Part print with two shaded views. Sizes in mm from the minimum x, y, z corner. A direction names the side the tool comes from. Round coordinates to 2 decimals unless told otherwise and drop trailing zeros. Loops run counter-clockwise (first coordinate to the right, second up) from the corner with the lowest first, then second, coordinate; pieces in that order, holes last. Notation, with made-up numbers: (-13.5, -4) -> (9.5, -4) arc R13 ccw to (9.5, 19) -> close; hole circle Ø9 at (54, -26.5). An arc over 180 degrees is marked (long way). Put each result on its own line as item: value. Start each with the question number.
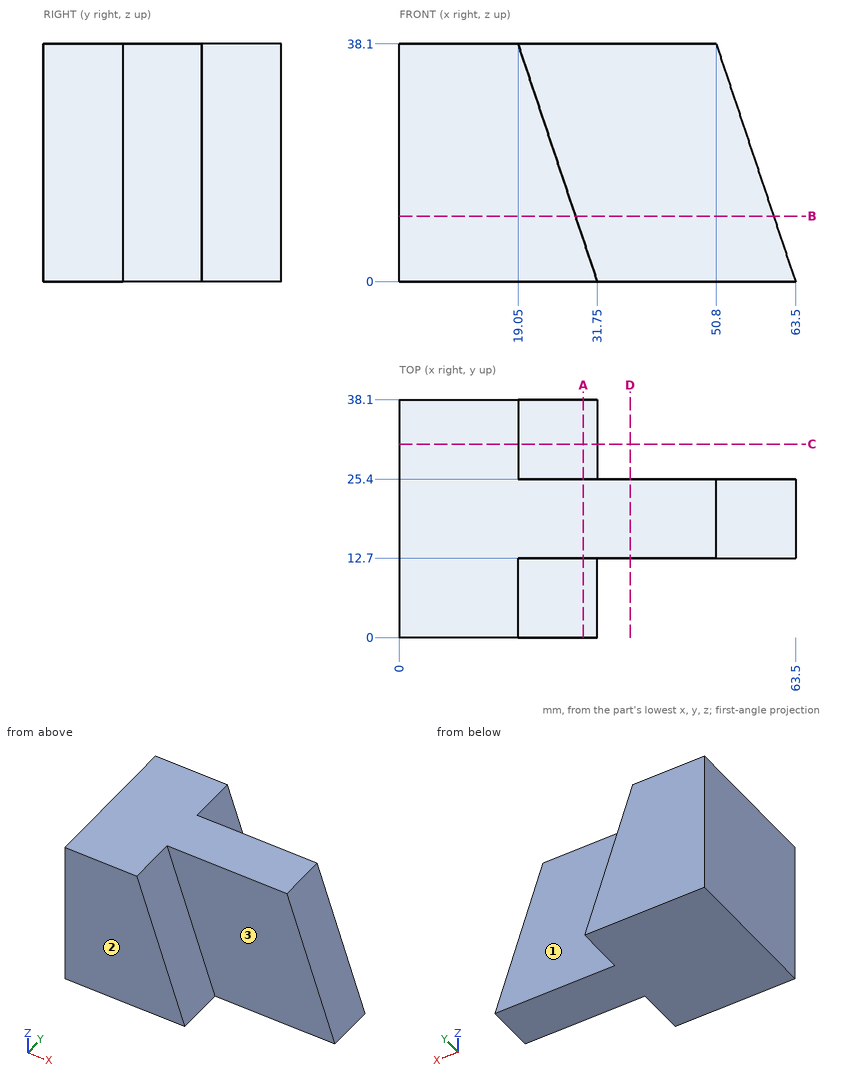
Item 1: Drop a flat-ended pin along its axis: pin 1 (2 mm diameter, centred on x = 40, z = 19.5, fed in from -Y). Give the stop position or say it passes through.
Item 2: Cut at A-A on x = 29.5. Write the cut outline in (y, z).
Item 3: Wall check: line 1 (Y direction, x = 48.5, z = 12.5); line 2 (X direction, y = 17.5, z = 25.5); line 3 (X direction, y = 16.5, z = 20). Give the ranges that are in metal, low to high. Write a range as from..to.
Item 4: 3-axis set-ups, long thin cutter, end or side, ignore diameter. For the marked faces 1, 2 and 3: which of +Z, -Z, +X, -X, +Y, -Y reach the whole face in a straight line?
Item 5: Cut at C-C on y = 31. Write the cut outline in (x, z), then the cut area to 3 significant figures.
Item 6: Cut at B-B on z = 10.5. Write the cut outline in (x, y).
Item 7: Cut at D-D on x = 37. Write the cut outline in (y, z), then the cut area to 3 significant figures.
Ans:
1. pin 1: stops at y = 12.7
2. outline: (0, 0) -> (38.1, 0) -> (38.1, 6.75) -> (25.4, 6.75) -> (25.4, 38.1) -> (12.7, 38.1) -> (12.7, 6.75) -> (0, 6.75) -> close
3. line 1: y = 12.7..25.4
3. line 2: x = 0..55
3. line 3: x = 0..56.83
4. face 1: +Z, +X, +Y
4. face 2: +Z, -Z, +X, -X, -Y
4. face 3: +Z, +X, -Y
5. outline: (0, 0) -> (31.75, 0) -> (19.05, 38.1) -> (0, 38.1) -> close
5. area: 968 mm2
6. outline: (0, 0) -> (28.25, 0) -> (28.25, 12.7) -> (60, 12.7) -> (60, 25.4) -> (28.25, 25.4) -> (28.25, 38.1) -> (0, 38.1) -> close
7. outline: (12.7, 0) -> (25.4, 0) -> (25.4, 38.1) -> (12.7, 38.1) -> close
7. area: 484 mm2
